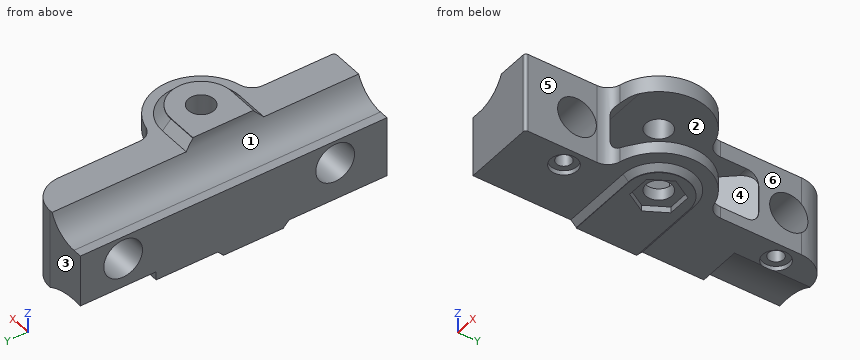
from build123d import *

# Parameters (mm, degrees)
SKETCH_R          = 4.25
PAD_DEPTH         = 28.5
PAD_DEPTH_BACK    = 5
FILLET_R          = 5
SKETCH002_R       = 6.4
POCKET_DEPTH      = 24.001
POCKET_DEPTH_BACK = -16.001
POCKET001_DEPTH   = 3
POCKET002_DEPTH   = 4
POCKET003_DEPTH   = 101.201
POCKET004_DEPTH   = 4
POCKET005_DEPTH   = 16
SKETCH028_R       = 22
POCKET006_DEPTH   = 25
SKETCH031_R       = 2.5
POCKET007_DEPTH   = 9
PAD001_DEPTH      = 17.2
SKETCH038_W       = 50
SKETCH038_H       = 26
POCKET008_DEPTH   = 2
SKETCH039_R       = 4.4
POCKET009_DEPTH   = 1.5
CHAMFER_SIZE      = 1.8
CHAMFER001_SIZE   = 2.8


with BuildPart() as part:
    # Sketch → Pad (new body, two sides)
    with BuildSketch(Plane.XY) as pad_sk:
        with BuildLine():
            ThreePointArc((0, -19), (16, -3), (0, 13))
            Line((0, 44.1), (0, 13))
            ThreePointArc((0, 44.1), (-2.928932, 51.171068), (-10, 54.1))
            Line((-24, 54.1), (-10, 54.1))
            Line((-24, 54.1), (-24, -47.1))
            Line((-24, -47.1), (-1, -47.1))
            ThreePointArc((-1, -47.1), (-0.292893, -46.807107), (0, -46.1))
            Line((0, -19), (0, -46.1))
        make_face()
        with Locations((0, -3)):
            Circle(SKETCH_R, mode=Mode.SUBTRACT)
    extrude(amount=PAD_DEPTH)
    extrude(pad_sk.sketch, amount=-PAD_DEPTH_BACK)

    # Fillet
    fillet_edges = [part.edges().sort_by_distance(p)[0] for p in [
        (0, 13, 11.75),
        (0, -19, 11.75),
    ]]
    fillet(fillet_edges, radius=FILLET_R)

    # Sketch002 → Pocket (cut, two sides)
    with BuildSketch(Plane.YZ) as pocket_sk:
        with Locations((-30, 11.5)):
            Circle(SKETCH002_R)
        with Locations((40, 11.5)):
            Circle(SKETCH002_R)
    extrude(amount=-POCKET_DEPTH, mode=Mode.SUBTRACT)
    extrude(pocket_sk.sketch, amount=-POCKET_DEPTH_BACK, mode=Mode.SUBTRACT)

    # Sketch013 → Pocket001 (cut)
    with BuildSketch(Plane.XY.offset(28.5)):
        with BuildLine():
            ThreePointArc((0, -13), (10, -3), (0, 7))
            Line((-40, 7), (0, 7))
            Line((-40, 7), (-40, 60))
            Line((-40, 60), (30, 60))
            Line((30, 60), (30, -60))
            Line((30, -60), (-40, -60))
            Line((-40, -60), (-40, -13))
            Line((-40, -13), (0, -13))
        make_face()
    extrude(amount=-POCKET001_DEPTH, mode=Mode.SUBTRACT)

    # Sketch024 → Pocket002 (cut)
    with BuildSketch(Plane(origin=(0, 0, -5), x_dir=(1, 0, 0), z_dir=(0, 0, -1))):
        with BuildLine():
            Line((0, 13), (-40, 13))
            Line((-40, 13), (-40, 65))
            Line((-40, 65), (24, 65))
            Line((24, 65), (24, -65))
            Line((24, -65), (-40, -65))
            Line((-40, -7), (-40, -65))
            Line((-40, -7), (0, -7))
            ThreePointArc((0, -7), (10, 3), (0, 13))
        make_face()
    extrude(amount=-POCKET002_DEPTH, mode=Mode.SUBTRACT)

    # Sketch029 → Pocket003 (cut, through all)
    with BuildSketch(Plane(origin=(0, 54.1, 0), x_dir=(-1, 0, 0), z_dir=(0, 1, 0))):
        with BuildLine():
            ThreePointArc((32, 30), (13.221825, 37.778175), (21, 19))
            Line((21, 19), (32, 19))
            Line((32, 30), (32, 19))
        make_face()
    extrude(amount=-POCKET003_DEPTH, mode=Mode.SUBTRACT)

    # Sketch027 → Pocket004 (cut)
    with BuildSketch(Plane(origin=(0, 0, -5), x_dir=(1, 0, 0), z_dir=(0, 0, -1))):
        Polygon((3.925982, 9.8), (-3.925982, 9.8), (-7.851964, 3), (-3.925982, -3.8), (3.925982, -3.8), (7.851964, 3), align=None)
    extrude(amount=-POCKET004_DEPTH, mode=Mode.SUBTRACT)

    # Sketch025 → Pocket005 (cut, symmetric)
    with BuildSketch(Plane.YZ):
        with BuildLine():
            Line((-16, 20.1), (26, 20.1))
            ThreePointArc((30, 16), (28.864001, 18.892928), (26, 20.1))
            Line((30, 16), (30, 7))
            ThreePointArc((26, 2.9), (28.864001, 4.107072), (30, 7))
            Line((26, 2.9), (-16, 2.9))
            ThreePointArc((-20, 7), (-18.864001, 4.107072), (-16, 2.9))
            Line((-20, 7), (-20, 16))
            ThreePointArc((-16, 20.1), (-18.864001, 18.892928), (-20, 16))
        make_face()
    extrude(amount=POCKET005_DEPTH, both=True, mode=Mode.SUBTRACT)

    # Sketch028 → Pocket006 (cut)
    with BuildSketch(Plane(origin=(0, 54.1, 0), x_dir=(-1, 0, 0), z_dir=(0, 1, 0))):
        with Locations((21, -20)):
            Circle(SKETCH028_R)
    extrude(amount=-POCKET006_DEPTH, mode=Mode.SUBTRACT)

    # Sketch031 → Pocket007 (cut)
    with BuildSketch(Plane(origin=(0, 0, -1), x_dir=(1, 0, 0), z_dir=(0, 0, -1))):
        with Locations((-6, 30)):
            Circle(SKETCH031_R)
        with Locations((-6, -40)):
            Circle(SKETCH031_R)
    extrude(amount=-POCKET007_DEPTH, mode=Mode.SUBTRACT)

    # Sketch032 → Pad001 (new body)
    with BuildSketch(Plane.XY.offset(2.9)):
        Polygon((0, -22), (-16, -11.5), (-16, -22), align=None)
        Polygon((-16, 12), (0, 30.1), (-16, 30.1), align=None)
    extrude(amount=PAD001_DEPTH)

    # Sketch038 → Pocket008 (cut)
    with BuildSketch(Plane(origin=(0, 0, -5), x_dir=(1, 0, 0), z_dir=(0, 0, -1))):
        with Locations((-10, 2)):
            Rectangle(SKETCH038_W, SKETCH038_H)
    extrude(amount=-POCKET008_DEPTH, mode=Mode.SUBTRACT)

    # Sketch039 → Pocket009 (cut)
    with BuildSketch(Plane(origin=(0, 0, -1), x_dir=(1, 0, 0), z_dir=(0, 0, -1))):
        with Locations((-6, 30)):
            Circle(SKETCH039_R)
        with Locations((-6, -40)):
            Circle(SKETCH039_R)
    extrude(amount=-POCKET009_DEPTH, mode=Mode.SUBTRACT)

    # Chamfer
    chamfer_edges = [part.edges().sort_by_distance(p)[0] for p in [
        (-12, -13, -1),
        (10, -3, -1),
        (-12, 7, -1),
    ]]
    chamfer(chamfer_edges, length=CHAMFER_SIZE)

    # Chamfer001
    chamfer001_edges = [part.edges().sort_by_distance(p)[0] for p in [
        (-5.481285, 7, 25.5),
        (10, -3, 25.5),
        (-5.481285, -13, 25.5),
    ]]
    chamfer(chamfer001_edges, length=CHAMFER001_SIZE)


solid = part.part
Build history of the part. All positions in model axes, mm. Face numbers are marked on the shaded views. A direction names the side the tool comes from. Round coordinates to 2 decimals unless told otherwise and drop trailing zeros. Write each loop counter-clockwise with the first axis right and the second up, starting at its lowest first coordinate (ties: lowest second). Pieces come first, ordered by that corner, then holes. Notation, with made-up numbers: M 8.25,16 L 21.25,16 A15 ccw 21.25,20 Z; hole C 14,20 d11. An arc over 180 degrees is marked long. Answer as a JSON object with one key per item and string values. Group by question number.
(1) Drill centre lines: L1, parallel to Y at x = -20, z = 11; L2, parallel to X at y = -30, z = 0.2; L3, parallel to Y at x = -21, z = 8. Where is each one in solid material? Low to high.
(2) Flat gauge pins, fed straight in: pin 1 (1.5 mm diameter, centred on y = 21.5, z = 19.5, fed in from +X); pin 2 (11.5 mm diameter, centred on x = -6, y = -30, fed in from -Z); pin 3 (5 mm diameter, centred on x = -1.5, z = 13.5, fed in from +Y); pin 4 (21.5 mm diameter, centred on x = 2.5, y = 11.5, fed in from +Z). Where does each tip first touch, or does it go through?
(3) Mould opens along Y. For the marked faces 1, 2 and 3 say: pulls with the +Y half, pulls with the -Y half, needs draft (parallel to the pull), parting line crosses it, or undercut.
(4) Cut at A-A (y = -30). Give the cut face in (x, z).
(5) Which spindle directions (+Z, -Z, +X, -X, +Y, -Y) get a long thin tool onto all of the face, cutting with end or side? Do the marked faces 4, 5 and 6. Say none if no direction does.
(6) Cut at D-D (y = 48). Give the cut face in (x, z), and give its area (3 significant figures).
(7) Cut at B-B (z = 11.5). Give the cut face in (x, y).
(8) Cut at C-C (x = -18.5). Give the cut face in (y, z), and give its area (3 significant figures).
Responses:
{
 "1": {"L1": "y = -47.1 to -36.38, -23.62 to 33.62, 46.38 to 54.1", "L2": "x = -24 to -10.4, -1.6 to 0", "L3": "y = -47.1 to -35.36, -24.64 to 34.64, 45.36 to 54.1"},
 "2": {"pin 1": "stops at x = 0", "pin 2": "stops at z = -1", "pin 3": "stops at y = 52.1", "pin 4": "stops at z = 28.5"},
 "3": {"face 1": "needs draft", "face 2": "undercut", "face 3": "pulls with the +Y half"},
 "4": {"outline": "M -24,-1 L -10.4,-1 L -10.4,0.5 L -8.5,0.5 L -8.5,5.1 L -24,5.1 Z; M -24,17.9 L 0,17.9 L 0,25.5 L -10.96,25.5 A11 cw -21,19 L -24,19 Z; M -3.5,0.5 L -1.6,0.5 L -1.6,-1 L 0,-1 L 0,5.1 L -3.5,5.1 Z"},
 "5": {"face 4": "+X", "face 5": "+Z, -Z, +X, -Y", "face 6": "+Z, -Z, +X, +Y"},
 "6": {"outline": "M -24,1.79 A22 cw -9.91,-1 L -0.79,-1 L -0.79,25.5 L -10.96,25.5 A11 cw -21,19 L -24,19 Z", "area": "517 mm2"},
 "7": {"outline": "M -24,-47.1 L -1,-47.1 A1 ccw 0,-46.1 L 0,-36.4 L -24,-36.4 Z; M -24,-23.6 L 0,-23.6 L 0,-23.4 A5 cw 1.33,-20 L -3.05,-20 L -16,-11.5 L -16,12 L -0.09,30 L 0,30 L 0,33.6 L -24,33.6 Z; M -24,46.4 L -0.27,46.4 A10 ccw -10,54.1 L -24,54.1 Z"},
 "8": {"outline": "M -47.1,-1 L -14.8,-1 L -13,-2.8 L -13,-3 L 7,-3 L 7,-2.8 L 8.8,-1 L 29.1,-1 L 29.1,1.86 L 54.1,1.86 L 54.1,19.29 L -47.1,19.29 Z; hole C -30,11.5 d12.8; hole C 40,11.5 d12.8", "area": "1,770 mm2"}
}
